Model file for the job. Use its own axes, mm. A direction names the side the tool comes from. Give positions to 0.01 mm unless a question says otherwise; leave off trailing zeros. Loops run counter-clockwise (first coordinate to the right, second up) from the corner with the lowest first, then second, coordinate; pieces in that order, holes last. Notation, with made-up numbers: M 78.25,-35 L 131.25,-35 A19 cw 131.25,-24 Z; hole C 5.25,41 d6. An arc over 180 degrees is marked long. Use CSV: the item, a comma, the result in double quotes. Start each with the question number.
(1) Tool access for faces 1 (the face through (-1.593, 6.219, -7.175)), 2 (the face through (2.3, 9, 4)), 3 (the face through (0, 9, 5.4)): list every direction of +Z, -Z, +X, -X, +Y, -Y with a clear straight run to the whole face (end or side of a thin tool).
(2) Two-plate mould, pull along Z, no slides. Class faces 4 (the face through (0, -1, -2)), 5 (the face through (-2.3, 9, -4)), 6 (the face through (-4, 9, -2.3)): pulls with the +Z half, pulls with the -Z half, needs draft (parallel to the pull), parting line crosses it, or undercut.
(3) Slice it at B-B on x = 0. List the corners of the cut face in (y, z), and give its area (3 significant figures).
(4) Wall check: line 1 along Z through (x, y) = (0, 7.4); line 2 along Z through (x, y) = (0, -1.15). Give the ranges that are in metal, low to high. Write a range as from..to.
(5) Slice it at D-D on y = 5. List the corners of the cut face in (x, z).
(6) Slice it at A-A on z = 0. List the corners of the cut face in (x, y), and give its area (3 significant figures).
(7) Flat gauge pins, fed straight in: P1, Ø3, axis at x = -2, y = 5, coming from the -Z side; P2, Ø3, axis at x = 0, z = 0, coming from the +Y side; P3, Ø2, axis at x = -4.5, y = 10, coming from the -Z side. Where does each tip first touch, or does it go through?
(8) Slice it at C-C on y = 7.25. List the corners of the cut face in (x, z), and give its area (3 significant figures).
Autodesk Inventor part; units mm, degrees
ref_plane "YZ Plane" through (0, 0, 0) normal (1, 0, 0) x (0, 1, 0)
ref_plane "XZ Plane" through (0, 0, 0) normal (0, 1, 0) x (-1, 0, 0)
ref_plane "XY Plane" through (0, 0, 0) normal (0, 0, 1) x (1, 0, 0)
sketch "Skizze1" plane through (0, 0, 0) normal (0, 1, 0) x (-1, 0, 0)
  circle A0 centre (0, 0) radius 10
  dimension "d0" = 20
extrude "Extrusion1" add sketch "Skizze1" along normal blind 2
sketch "Skizze2" plane through (0, 2, 0) normal (0, 1, 0) x (1, 0, 0)
  circle A0 centre (0, 0) radius 9
  dimension "d3" = 18
extrude "Extrusion2" add sketch "Skizze2" along normal blind 2
sketch "Skizze3" plane through (0, 4, 0) normal (0, 1, 0) x (1, 0, 0)
  circle A0 centre (0, 0) radius 7.35
  dimension "d6" = 14.7
extrude "Extrusion3" add sketch "Skizze3" along normal blind 4.5
sketch "Skizze4" plane through (0, 8.5, 0) normal (0, 1, 0) x (1, 0, 0)
  line L0 (-5.4, 5.4) -> (5.4, 5.4)
  line L1 (5.4, 5.4) -> (5.4, -5.4)
  line L2 (5.4, -5.4) -> (-5.4, -5.4)
  line L3 (-5.4, -5.4) -> (-5.4, 5.4)
  line L4 (0, 14) -> (0, -14)
  line L5 (-14, 0) -> (14, 0)
  line L6 (-5.4, 5.4) -> (-2.3, 5.4)
  line L7 (-2.3, 5.4) -> (-2.3, 2.3)
  line L8 (-2.3, 2.3) -> (-5.4, 2.3)
  line L9 (-5.4, 2.3) -> (-5.4, 5.4)
  line L10 (5.4, 5.4) -> (2.3, 5.4)
  line L11 (2.3, 5.4) -> (2.3, 2.3)
  line L12 (2.3, 2.3) -> (5.4, 2.3)
  line L13 (5.4, 2.3) -> (5.4, 5.4)
  line L14 (5.4, -5.4) -> (2.3, -5.4)
  line L15 (2.3, -5.4) -> (2.3, -2.3)
  line L16 (2.3, -2.3) -> (5.4, -2.3)
  line L17 (5.4, -2.3) -> (5.4, -5.4)
  line L18 (-5.4, -5.4) -> (-2.3, -5.4)
  line L19 (-2.3, -5.4) -> (-2.3, -2.3)
  line L20 (-2.3, -2.3) -> (-5.4, -2.3)
  line L21 (-5.4, -2.3) -> (-5.4, -5.4)
  point P0 (0, 0)
  point P1 (5.4, 2.3)
  point P2 (-5.4, 2.3)
  point P3 (-5.4, -2.3)
  point P4 (2.3, -5.4)
  point P5 (5.4, -2.3)
  dimension "d9" = 10.8
  dimension "d10" = 10.8
  dimension "d11" = 3.1
  dimension "d12" = 3.1
  dimension "d13" = 3.1
  dimension "d14" = 3.1
  dimension "d15" = 3.1
  dimension "d16" = 3.1
  dimension "d17" = 3.1
  dimension "d18" = 3.1
extrude "Extrusion4" add sketch "Skizze4" along normal blind 2 contours L0 L4 L5 L3 L8 L7 | L0 L11 L12 L1 L5 L4 | L5 L4 L2 L19 L20 L3 | L5 L1 L16 L15 L2 L4
sketch "Skizze5" plane through (0, 10.5, 0) normal (0, 1, 0) x (1, 0, 0)
  circle A0 centre (0, 0) radius 2
  dimension "d21" = 4
extrude "Extrusion5" cut sketch "Skizze5" against normal blind 5
sketch "Skizze6" plane through (0, 0, 0) normal (0, -1, 0) x (1, 0, 0)
  line L0 (-12.5, 12.5) -> (12.5, 12.5)
  line L1 (12.5, 12.5) -> (12.5, -12.5)
  line L2 (12.5, -12.5) -> (-12.5, -12.5)
  line L3 (-12.5, -12.5) -> (-12.5, 12.5)
  line L4 (-12.5, 12.5) -> (12.5, -12.5) construction
  line L5 (12.5, 12.5) -> (-12.5, -12.5) construction
  point P0 (0, 0)
  dimension "d24" = 25
  dimension "d25" = 25
extrude "Extrusion6" add sketch "Skizze6" along normal blind 3
sketch "Skizze7" plane through (0, -3, 0) normal (0, -1, 0) x (1, 0, 0)
  circle A0 centre (0, 0) radius 2
  dimension "d28" = 4
extrude "Extrusion7" cut sketch "Skizze7" against normal blind 5
properties part number "_3D-Druck"
Reply:
1,face 1,"+Y"
1,face 2,"+Z, +X, +Y"
1,face 3,"+Z, +X, -X, +Y"
2,face 4,"undercut"
2,face 5,"needs draft"
2,face 6,"pulls with the -Z half"
3,outline,"M -3,-12.5 L 0,-12.5 L 0,-10 L 2,-10 L 2,-9 L 4,-9 L 4,-7.35 L 8.5,-7.35 L 8.5,-5.4 L 10.5,-5.4 L 10.5,-2 L 5.5,-2 L 5.5,2 L 10.5,2 L 10.5,5.4 L 8.5,5.4 L 8.5,7.35 L 4,7.35 L 4,9 L 2,9 L 2,10 L 0,10 L 0,12.5 L -3,12.5 L -3,2 L 2,2 L 2,-2 L -3,-2 Z"
3,area,"199 mm^2"
4,line 1,"z = -7.35..-2, 2..7.35"
4,line 2,"z = -12.5..-2, 2..12.5"
5,outline,"C 0,0 d14.7"
6,outline,"M -12.5,-3 L -2,-3 L -2,2 L 2,2 L 2,-3 L 12.5,-3 L 12.5,0 L 10,0 L 10,2 L 9,2 L 9,4 L 7.35,4 L 7.35,8.5 L 5.4,8.5 L 5.4,10.5 L 2,10.5 L 2,5.5 L -2,5.5 L -2,10.5 L -5.4,10.5 L -5.4,8.5 L -7.35,8.5 L -7.35,4 L -9,4 L -9,2 L -10,2 L -10,0 L -12.5,0 Z"
6,area,"199 mm^2"
7,P1,"stops at z = -8.96"
7,P2,"stops at y = 5.5"
7,P3,"stops at z = -2.3"
8,outline,"C 0,0 d14.7; hole C 0,0 d4"
8,area,"157 mm^2"
